Verification items for the finished model (mm, model axes). A direction names the side the tool comes from. Coordinates: 2 decimals unless noted, no trailing zeros. Order: outer loops, then holes, each group sorted by start corner. A loop starts at its lowest first (then second) coordinate and runs counter-clockwise, first axis right, second up.
Q1. Cross-section at D-D, the plane y = -3.5. Record the boundary of the cut face in (x, z).
Q2. Draft check along X on faces 1 (the flat face through (45, 6, -27.67)), 2 (the flat face through (-51.5, -5, 17)), 3 (the flat face through (43.28, 6, -27)). Enter one of: pulls with the +X half, pulls with the -X half, needs draft (parallel to the pull), parting line crosses it, or undercut.
Q3. Cross-section at C-C, the plane z = 18. Record the boundary of the cut face in (x, y), and give its area (3 significant figures).
Q4. Depth check by flat-ended pin: P1, Ø3, axis at x = 32, z = -7, coming from the +Y side; P2, Ø1, axis at y = 7.5, z = -27, coming from the +X side; P3, Ø3, axis at y = 8, z = -26.5, coming from the -X side; P4, Ø10, axis at y = 6.5, z = 12, coming from the -X side. Enter the tip coordinate at first touch or a pass-through.
Q5. Cross-section at A-A, the plane y = 6.5. Record the boundary of the cut face in (x, z), and give its area (3 significant figures).
Q6. Thickness scan on line 1 (Z direction, x = -8.5, y = 3); line 2 (Y direction, x = -27.5, z = 19.5); line 3 (Y direction, x = 9.5, z = -27). Record the ranges inside material, lowest first.
Q7. Set-up check for faces 4 (the flat face through (-47, -5, 14.34)), 5 (the flat face through (45, 6, -25.67)), 6 (the flat face through (-47, -5, 20.34)), 7 (the flat face through (-16, 6, -24.17)), 8 (the flat face through (15.68, 6, 26)): record each of +Z, -Z, +X, -X, +Y, -Y from which the full face is reachable in a straight line by a thin tool's end or side.
Q8. Cross-section at B-B, the plane x = -30. Record the boundary of the cut face in (y, z), and give its area (3 significant figures).
from build123d import *

# Parameters (mm, degrees)
SKETCH2_W           = 97
SKETCH2_H           = 66
BOSS_EXTRUDE2_DEPTH = 1
SKETCH3_W           = 62.96
SKETCH3_H           = 3.5
BOSS_EXTRUDE3_DEPTH = 10
SKETCH4_W           = 9
SKETCH4_H           = 6
BOSS_EXTRUDE4_DEPTH = 10
SKETCH5_W           = 4
SKETCH5_H           = 2
BOSS_EXTRUDE5_DEPTH = 10


with BuildPart() as part:
    # Sketch2 → Boss-Extrude2 (new body)
    with BuildSketch(Plane(origin=(0, 0, 0), x_dir=(1, 0, 0), z_dir=(0, 1, 0))):
        Rectangle(SKETCH2_W, SKETCH2_H)
    extrude(amount=BOSS_EXTRUDE2_DEPTH)

    # Sketch3 → Boss-Extrude3 (add)
    with BuildSketch(Plane(origin=(0, 1, 0), x_dir=(1, 0, 0), z_dir=(0, 1, 0))):
        with Locations((-15.8, 25.92)):
            Rectangle(SKETCH3_W, SKETCH3_H)
        with Locations((-15.8, -25.92)):
            Rectangle(SKETCH3_W, SKETCH3_H)
    extrude(amount=BOSS_EXTRUDE3_DEPTH)

    # Sketch4 → Boss-Extrude4 (add)
    with BuildSketch(Plane.XZ):
        with Locations((-47, 17.34)):
            Rectangle(SKETCH4_W, SKETCH4_H)
    extrude(amount=BOSS_EXTRUDE4_DEPTH)

    # Sketch5 → Boss-Extrude5 (add)
    with BuildSketch(Plane(origin=(0, 1, 0), x_dir=(1, 0, 0), z_dir=(0, 1, 0))):
        with Locations((45.28, 26.67)):
            Rectangle(SKETCH5_W, SKETCH5_H)
        with Locations((45.28, -26.67)):
            Rectangle(SKETCH5_W, SKETCH5_H)
    extrude(amount=BOSS_EXTRUDE5_DEPTH)


solid = part.part
Check values:
1. outline: (-51.5, 14.34) - (-42.5, 14.34) - (-42.5, 20.34) - (-51.5, 20.34) - close
2. face 1: needs draft
2. face 2: pulls with the -X half
2. face 3: undercut
3. outline: (-51.5, -10) - (-42.5, -10) - (-42.5, 0) - (48.5, 0) - (48.5, 1) - (-48.5, 1) - (-48.5, 0) - (-51.5, 0) - close
3. area: 187 mm2
4. P1: stops at y = 1
4. P2: stops at x = 47.28
4. P3: stops at x = -47.28
4. P4: passes through
5. outline: (-47.28, -27.67) - (15.68, -27.67) - (15.68, -24.17) - (-47.28, -24.17) - close; (-47.28, 24.17) - (15.68, 24.17) - (15.68, 27.67) - (-47.28, 27.67) - close; (43.28, -27.67) - (47.28, -27.67) - (47.28, -25.67) - (43.28, -25.67) - close; (43.28, 25.67) - (47.28, 25.67) - (47.28, 27.67) - (43.28, 27.67) - close
5. area: 457 mm2
6. line 1: z = -27.67 to -24.17, 24.17 to 27.67
6. line 2: y = 0 to 1
6. line 3: y = 0 to 11
7. face 4: -Z, +X, -X, -Y
7. face 5: +X, +Y
7. face 6: +Z, +X, -X, -Y
7. face 7: +X, -X, +Y
7. face 8: +Z, -Z, +Y
8. outline: (0, -33) - (1, -33) - (1, -27.67) - (11, -27.67) - (11, -24.17) - (1, -24.17) - (1, 24.17) - (11, 24.17) - (11, 27.67) - (1, 27.67) - (1, 33) - (0, 33) - close
8. area: 136 mm2
